Build history of the part. All positions in model axes, mm. A direction names the side the tool comes from. Round coordinates to 2 decimals unless told otherwise and drop trailing zeros. Loops run counter-clockwise (first coordinate to the right, second up) from the corner with the lowest first, then second, coordinate; pieces in that order, holes last. Notation, with made-up numbers: (-10, 15) - (40, 15) arc R19 cw to (40, 41) - close; hole circle Ø10 at (53.5, 27.5). An arc over 180 degrees is marked (long way). One line per question, with ' | ' between items. Start each with the question number.
from build123d import *

# Parameters (mm, degrees)
SKETCH1_R             = 1.25
BOSS_EXTRUDE1_DEPTH   = 4.5
BOSS_EXTRUDE2_START   = -3.5
BOSS_EXTRUDE2_DEPTH   = 1
SKETCH3_W             = 2
SKETCH3_H             = 3.5
BOSS_EXTRUDE3_DEPTH   = 4.75
FILLET2_R             = 0.5
F_2_0MM_DOWEL_HOLE1_D = 2
CHAMFER1_SIZE         = 0.25


with BuildPart() as part:
    # Sketch1 → Boss-Extrude1 (new body, symmetric)
    with BuildSketch(Plane(origin=(0, 0, 0), x_dir=(1, 0, 0), z_dir=(0, 1, 0))):
        Circle(SKETCH1_R)
    extrude(amount=BOSS_EXTRUDE1_DEPTH, both=True)

    # Sketch2 → Boss-Extrude2 (add)
    with BuildSketch(Plane(origin=(0, 0, 0), x_dir=(1, 0, 0), z_dir=(0, 1, 0)).offset(BOSS_EXTRUDE2_START)):
        with BuildLine():
            Line((-2, -1), (-2, 1))
            ThreePointArc((-2, 1), (0, 1.75), (2, 1))
            Line((2, 1), (2, -1))
            ThreePointArc((2, -1), (0, -1.75), (-2, -1))
        make_face()
    boss_extrude2 = extrude(amount=-BOSS_EXTRUDE2_DEPTH)

    # Mirror2: Boss-Extrude2 across plane
    add(boss_extrude2.mirror(Plane.ZX))

    # Sketch3 → Boss-Extrude3 (add, symmetric)
    with BuildSketch(Plane(origin=(0, 0, 0), x_dir=(1, 0, 0), z_dir=(0, 1, 0))):
        with Locations((-3, 0)):
            Rectangle(SKETCH3_W, SKETCH3_H)
    boss_extrude3 = extrude(amount=BOSS_EXTRUDE3_DEPTH, both=True)

    # Mirror3: Boss-Extrude3 across plane
    add(boss_extrude3.mirror(Plane(origin=(0, 0, 0), x_dir=(0, 0, 1), z_dir=(1, 0, 0))))

    # Fillet2
    fillet2_edges = [part.edges().sort_by_distance(p)[0] for p in [
        (-2, 0, 1.75),
        (-4, 0, -1.75),
        (-4, 0, 1.75),
        (-2, 0, -1.75),
        (2, 0, -1.75),
        (4, 0, 1.75),
        (4, 0, -1.75),
        (2, 0, 1.75),
    ]]
    fillet(fillet2_edges, radius=FILLET2_R)

    # Ø2.0mm Dowel Hole1 (through all)
    with Locations(Plane(origin=(0, 4.5, 0), x_dir=(1, 0, 0), z_dir=(0, 1, 0))):
        with Locations((0, 0)):
            Hole(F_2_0MM_DOWEL_HOLE1_D / 2)

    # Chamfer1
    chamfer1_edges = [part.edges().sort_by_distance(p)[0] for p in [
        (1, -4.5, 0),
        (1, 4.5, 0),
    ]]
    chamfer(chamfer1_edges, length=CHAMFER1_SIZE)


solid = part.part
1) Saw through at B-B on z = 0. Write the cut outline in (x, y), and give its area (3 significant figures).
2) Drop flat-ended pins along their axis: pin 1 (3 mm diameter, centred on x = -2, y = -1, fed in from +Z); pin 2 (1.7 mm diameter, centred on x = -0.5, z = 1, fed in from -Y). Give the stop position or say it passes through.
3) Wall check: line 1 (X direction, y = 1.25, z = 0); line 2 (Z direction, x = 0, y = -0.25); line 3 (X direction, y = -2, z = -1.1). Give the ranges that are in metal, low to high. Write a range as [from, to].
4) Saw through at C-C on x = 0. Write the cut outline in (y, z), and give its area (4 significant figures).
5) Tool access for faces 1 (the cylindrical face through (-0.27, 0.05, 1.22)), 2 (the cylindrical face through (0, 0, 1)): list every direction of +Z, -Z, +X, -X, +Y, -Y with a clear straight run to the whole face (end or side of a thin tool).
6) Saw through at D-D on x = 1.5. Write the cut outline in (y, z).
7) Two-plate mould, pull along Y, no slides. Class faces 3 (the flat face through (2, 0, 0)), 4 (the flat face through (4, 0, 0)), 5 (the flat face through (3, 4.75, 0)): +Y half, -Y half, draft (parallel to the pull), parting line (faces both ways), or undercut.
8) Saw through at A-A on y = -3. Write the cut outline in (x, z), and give its area (3 significant figures).
Answer key:
1) outline: (-4, -4.75) - (-2, -4.75) - (-2, -4.5) - (-1.25, -4.5) - (-1, -4.25) - (-1, 4.25) - (-1.25, 4.5) - (-2, 4.5) - (-2, 4.75) - (-4, 4.75) - close; (1, -4.25) - (1.25, -4.5) - (2, -4.5) - (2, -4.75) - (4, -4.75) - (4, 4.75) - (2, 4.75) - (2, 4.5) - (1.25, 4.5) - (1, 4.25) - close; hole (-2, -3.5) - (-1.25, -3.5) - (-1.25, 3.5) - (-2, 3.5) - close; hole (1.25, -3.5) - (2, -3.5) - (2, 3.5) - (1.25, 3.5) - close | area: 45.4 mm²
2) pin 1: z = 1.75 | pin 2: y = -4.5
3) line 1: [-4, -2], [-1.25, -1], [1, 1.25], [2, 4] | line 2: [-1.25, -1], [1, 1.25] | line 3: [-4, -2], [-0.59, 0.59], [2, 4]
4) outline: (-4.5, -1.75) - (-3.5, -1.75) - (-3.5, -1.25) - (3.5, -1.25) - (3.5, -1.75) - (4.5, -1.75) - (4.5, -1.25) - (4.25, -1) - (-4.25, -1) - (-4.5, -1.25) - close; (-4.5, 1.25) - (-4.25, 1) - (4.25, 1) - (4.5, 1.25) - (4.5, 1.75) - (3.5, 1.75) - (3.5, 1.25) - (-3.5, 1.25) - (-3.5, 1.75) - (-4.5, 1.75) - close | area: 6.375 mm²
5) face 1: none | face 2: +Y, -Y
6) outline: (-4.5, -1.35) - (-3.5, -1.35) - (-3.5, 1.35) - (-4.5, 1.35) - close; (3.5, -1.35) - (4.5, -1.35) - (4.5, 1.35) - (3.5, 1.35) - close
7) face 3: undercut | face 4: draft | face 5: +Y half
8) outline: (-4, -1.25) arc R0.5 ccw to (-3.5, -1.75) - (-2.5, -1.75) arc R0.5 ccw to (-2, -1.25) - (-2, 1.25) arc R0.5 ccw to (-2.5, 1.75) - (-3.5, 1.75) arc R0.5 ccw to (-4, 1.25) - close; circle Ø2.5 at (0, 0); (2, -1.25) arc R0.5 ccw to (2.5, -1.75) - (3.5, -1.75) arc R0.5 ccw to (4, -1.25) - (4, 1.25) arc R0.5 ccw to (3.5, 1.75) - (2.5, 1.75) arc R0.5 ccw to (2, 1.25) - close; hole circle Ø2 at (0, 0) | area: 15.3 mm²
